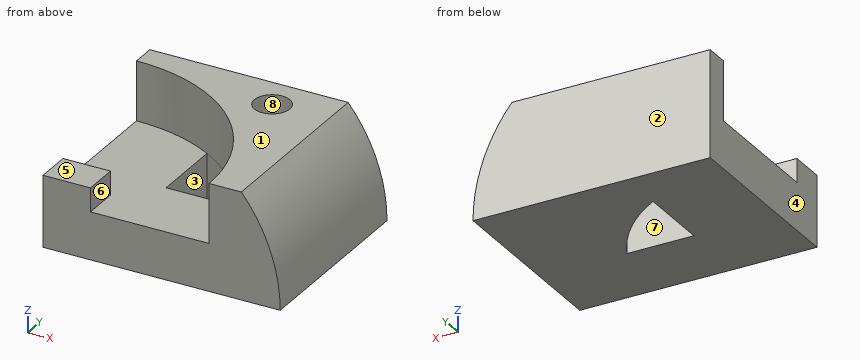
from build123d import *

# Parameters (mm, degrees)
F1_DEPTH  = 80
F3_R      = 70
F4_DEPTH  = 25
F5_W      = 20
F5_H      = 15
F6_DEPTH  = 10
F8_DEPTH  = 20.001
F10_R     = 7.5
F11_DEPTH = 30


with BuildPart() as f1:
    # F0 (on Front) → F1 (new body)
    with BuildSketch(Plane.XZ):
        with BuildLine():
            Line((0, 0), (100, 0))
            ThreePointArc((100, 0), (95.777397, 23.944395), (83.619026, 45))
            Line((83.619026, 45), (0, 45))
            Line((0, 45), (0, 0))
        make_face()
    extrude(amount=F1_DEPTH)

    # F3 (on face) → F4 (cut, through all)
    with BuildSketch(Plane.XY.offset(45)):
        with Locations((0, -80)):
            Circle(F3_R)
    extrude(amount=-F4_DEPTH, mode=Mode.SUBTRACT)

    # F5 (on face) → F6 (join)
    with BuildSketch(Plane.XY.offset(20)):
        with Locations((10, -72.5)):
            Rectangle(F5_W, F5_H)
    extrude(amount=F6_DEPTH)

    # F7 (on face) → F8 (cut, through all)
    with BuildSketch(Plane.XY.offset(20)):
        with BuildLine():
            ThreePointArc((63.245553, -50), (51.453576, -32.539179), (35, -19.378222))
            Line((35, -19.378222), (35, -50))
            Line((35, -50), (63.245553, -50))
        make_face()
    extrude(amount=-F8_DEPTH, mode=Mode.SUBTRACT)

    # F10 (on face) → F11 (cut, through all)
    with BuildSketch(Plane.XY.offset(45)):
        with Locations((60, -15)):
            Circle(F10_R)
    extrude(amount=-F11_DEPTH, mode=Mode.SUBTRACT)


solid = f1.part
Can you work these out from the model? Positions are in its coordinate system, mm. Face numbers are marked on the shaded views. A direction names the side the tool comes from. Give positions to 0.01 mm unless a question says otherwise; leave off trailing zeros. Write each loop counter-clockwise with the first axis right and the second up, starting at its lowest first coordinate (ties: lowest second). Pieces come first, ordered by that corner, then holes. Notation, with made-up numbers: (-30.75, 62) -> (2.25, 62) arc R9 cw to (2.25, 72) -> close; hole circle Ø8 at (-30.75, 16). An arc over 180 degrees is marked (long way). Answer as a JSON object with one key per item and string values. Group by question number.
Item 1: I'm going to push flat-ended pins straight in: P1, Ø10, axis at y = -30, z = 9.5, coming from the +X side; P2, Ø6, axis at y = -71, z = 4.5, coming from the +X side; P3, Ø8, axis at y = -73.5, z = 24.5, coming from the +X side. Where does each tip first touch, or does it pass through?
Item 2: Suppose I cut it at C-C (z = 5). Please give me the cut outline in (x, y), plus the area to 3 significant figures.
Item 3: Please list where these lines run through material, in increasing order: line 1 (Z direction, x = 6, y = -36); line 2 (Y direction, x = 60, z = 37); line 3 (Y direction, x = 9, z = 27). Write a range as [from, to].
Item 4: Suppose I cut it at D-D (y = -15). Please give me the cut outline in (x, z).
Item 5: Suppose I cut it at B-B (y = -36.5). Please give me the cut outline in (x, z), plus the area to 3 significant figures.
Item 6: Suppose I cut it at A-A (x = 48.5). Please give me the cut outline in (y, z), plus the area to 3 significant figures.
Item 7: We'd pull the mould along Y, two halves only. Please class the marked faces 1, 2 and 3: +Y half, -Y half, draft (parallel to the pull), parting line (faces both ways), or undercut.
Item 8: For the marked faces 4, 5, 6, 7 and 8, which set-ups out of +Z, -Z, +X, -X, +Y, -Y let a thin tool reach every point of the face, with its end or its side?
Findings:
{
 "1": {"P1": "stops at x = 99.86", "P2": "stops at x = 99.98", "P3": "stops at x = 96.93"},
 "2": {"outline": "(0, -80) -> (99.82, -80) -> (99.82, 0) -> (0, 0) -> close; hole (35, -50) -> (63.25, -50) arc R70 ccw to (35, -19.38) -> close", "area": "7,460 mm²"},
 "3": {"line 1": "z = [0, 20]", "line 2": "y = [-43.94, -22.5], [-7.5, 0]", "line 3": "y = [-80, -65], [-10.58, 0]"},
 "4": {"outline": "(0, 0) -> (100, 0) arc R70 ccw to (83.62, 45) -> (67.5, 45) -> (67.5, 15) -> (52.5, 15) -> (52.5, 45) -> (25.98, 45) -> (25.98, 20) -> (0, 20) -> close"},
 "5": {"outline": "(0, 0) -> (35, 0) -> (35, 20) -> (0, 20) -> close; (54.84, 0) -> (100, 0) arc R70 ccw to (83.62, 45) -> (54.84, 45) -> close", "area": "2,500 mm²"},
 "6": {"outline": "(-80, 0) -> (-50, 0) -> (-50, 20) -> (-80, 20) -> close; (-29.52, 0) -> (0, 0) -> (0, 45) -> (-29.52, 45) -> close", "area": "1,930 mm²"},
 "7": {"face 1": "draft", "face 2": "+Y half", "face 3": "undercut"},
 "8": {"face 4": "+Z, -Z, -X, +Y, -Y", "face 5": "+Z, -X, -Y", "face 6": "+Z, -Y", "face 7": "+Z, -Z", "face 8": "+Z"}
}
